Part model, mm, in its own coordinate system. Face numbers are marked on the shaded views. A direction names the side the tool comes from. Round coordinates to 2 decimals unless told otherwise and drop trailing zeros. Write each loop counter-clockwise with the first axis right and the second up, starting at its lowest first coordinate (ties: lowest second). Pieces come first, ordered by that corner, then holes. Notation, with made-up numbers: M -39.5,82.25 L -12.5,82.25 A27 cw -12.5,116.25 Z; hole C 46,84 d1. An arc over 180 degrees is marked long. Use a Markdown table: item, result. Add a question column.
1) Two-plate mould, pull along X, no slides. Class the marked faces 3, 4 and 5: released by +X, released by -X, zero draft, split by the parting line, or undercut.
2) Slice it at C-C on x = 21.5. Write the cut outline in (y, z), plus the area to 3 significant figures.
3) Wall check: probe 1 along X at (y, z) = (-18, 23.5); probe 2 along Z at (x, y) = (187, -21.5); probe 3 along X at (y, z) = (-26.5, 4). Give the ranges that are in metal, low to high.
4) Slice it at A-A on z = 20. Write the cut outline in (x, y).
5) Which spindle directions (+Z, -Z, +X, -X, +Y, -Y) get a long thin tool onto all of the face, cutting with end or side? Do the marked faces 1 and 2. Say none if no direction does.
6) Slice it at B-B on y = -37. Write the cut outline in (x, z) (3 decimals), plus the area to 3 significant figures.
7) Drop a flat-ended pin along its axis: P1, Ø10, axis at x = 37.5, y = -16.5, coming from the +Z side. Give the stop position or say it passes through.
Autodesk Inventor part; units mm, degrees
ref_plane "YZ Plane" through (0, 0, 0) normal (1, 0, 0) x (0, 1, 0)
ref_plane "XZ Plane" through (0, 0, 0) normal (0, 1, 0) x (-1, 0, 0)
ref_plane "XY Plane" through (0, 0, 0) normal (0, 0, 1) x (1, 0, 0)
sketch "Sketch1" plane through (0, 0, 0) normal (0, 0, 1) x (1, 0, 0)
  line L0 (0, 0) -> (304.8, 0)
  line L1 (304.8, 0) -> (304.8, -50.8)
  line L2 (304.8, -50.8) -> (0, -50.8)
  line L3 (0, -50.8) -> (0, 0)
  dimension "d0" = 304.8
  dimension "d1" = 50.8
extrude "Extrusion1" add sketch "Sketch1" along normal blind 2.2098
sketch "Sketch2" plane through (0, 0, 2.2098) normal (0, 0, 1) x (1, 0, 0)
  line L0 (0, -50.8) -> (304.8, -50.8)
  line L1 (0, 0) -> (2.2098, 0)
  line L2 (2.2098, 0) -> (2.2098, -50.8)
  line L3 (2.2098, -50.8) -> (0, -50.8)
  line L4 (0, -50.8) -> (0, 0)
  line L5 (304.8, 0) -> (302.5902, 0)
  line L6 (302.5902, 0) -> (302.5902, -50.8)
  line L7 (302.5902, -50.8) -> (304.8, -50.8)
  line L8 (304.8, -50.8) -> (304.8, 0)
  dimension "d4" = 2.2098
  dimension "d5" = 2.2098
extrude "Extrusion2" add sketch "Sketch2" along normal blind 50.8
fillet "Fillet1" radius 3.175 1 edges at (304.8, -25.4, 0)
fillet "Fillet2" radius 3.175 1 edges at (0, -25.4, 0)
fillet "Fillet3" radius 3.175 1 edges at (2.2098, -25.4, 2.2098)
fillet "Fillet4" radius 3.175 1 edges at (302.5902, -25.4, 2.2098)
properties part number "Conveyor Brace"
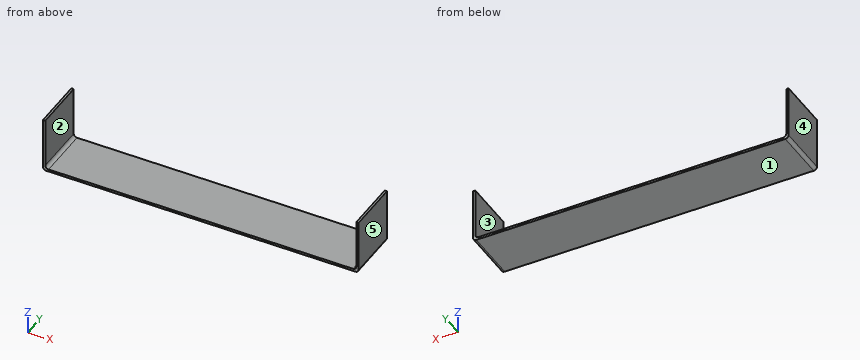
Entries:
| question | item | result |
|---|---|---|
| 1 | face 3 | undercut |
| 1 | face 4 | released by -X |
| 1 | face 5 | released by +X |
| 2 | outline | M -50.8,0 L 0,0 L 0,2.21 L -50.8,2.21 Z |
| 2 | area | 112 mm^2 |
| 3 | probe 1 | x = 0 to 2.21, 302.59 to 304.8 |
| 3 | probe 2 | z = 0 to 2.21 |
| 3 | probe 3 | x = 0 to 2.53, 302.27 to 304.8 |
| 4 | outline | M 0,-50.8 L 2.21,-50.8 L 2.21,0 L 0,0 Z; M 302.59,-50.8 L 304.8,-50.8 L 304.8,0 L 302.59,0 Z |
| 5 | face 1 | -Z, +X, -X, +Y, -Y |
| 5 | face 2 | +Z, +Y, -Y |
| 6 | outline | M 0,3.175 A3.175 ccw 3.175,0 L 301.625,0 A3.175 ccw 304.8,3.175 L 304.8,53.01 L 302.59,53.01 L 302.59,5.385 A3.175 cw 299.415,2.21 L 5.385,2.21 A3.175 cw 2.21,5.385 L 2.21,53.01 L 0,53.01 Z |
| 6 | area | 898 mm^2 |
| 7 | P1 | stops at z = 2.21 |
